The model under review builds one solid part; all positions refer to its coordinate system, in mm. Coordinates: 2 decimals unless noted, no trailing zeros. Write each loop counter-clockwise with the first axis right and the second up, starting at its lowest first coordinate (ties: lowest second). Pieces come first, ordered by that corner, then holes. Notation, with made-up numbers: (27.5, -27.5) - (74.5, -27.5) arc R17 ccw to (74.5, -15.5) - close; hole circle Ø10 at (28, 71.25). An arc over 180 degrees is marked (long way). Put each result on its own line as item: value. Start each with the question number.
Item 1: To check wall thickness, follow L1, parallel to X at y = 2.7, z = 89; L2, parallel to X at y = 1.85, z = 3.5; L3, parallel to Z at x = -77.5, y = 1.85. State the ranges of each line that lie inside material, in increasing order. Write a range as [from, to].
Item 2: For pin 1 (4 mm diameter, centred on x = -82.03, z = 105.37, fed in from +Y); pin 2 (1.8 mm diameter, centred on x = 64.34, z = 87.67, fed in from +Y); pin 3 (1.5 mm diameter, centred on y = 0.5, z = -130.5, fed in from -X); pin 4 (1.5 mm diameter, centred on y = 2, z = -53, fed in from -X), all flat-tipped, find the tip position at first contact; note any pin that passes through.
Item 3: Consider section B-B on z = 167. Give the boundary of the cut face in (x, y).
Item 4: Consider section C-C on x = -133. Give the boundary of the cut face in (y, z).
Item 5: Consider section A-A on y = 1.55. State how many separate pieces and enclosed holes the cut face has, then the cut area to 3 significant figures.
```python
from build123d import *

# Parameters (mm, degrees)
SKETCH1_R           = 200
BOSS_EXTRUDE1_DEPTH = 3
CUT_EXTRUDE1_DEPTH  = 3
SKETCH3_R           = 75
CUT_EXTRUDE2_DEPTH  = 10
SKETCH5_R           = 1.5
CUT_EXTRUDE4_DEPTH  = 73


with BuildPart() as part:
    # Sketch1 → Boss-Extrude1 (new body)
    with BuildSketch(Plane(origin=(0, 0, 0), x_dir=(1, 0, 0), z_dir=(0, 1, 0))):
        with Locations(Location((0, 0, 0), (0, 0, 270))):
            Circle(SKETCH1_R)
    extrude(amount=BOSS_EXTRUDE1_DEPTH)

    # Sketch2 → Cut-Extrude1 (cut)
    with BuildSketch(Plane(origin=(0, 3, 0), x_dir=(1, 0, 0), z_dir=(0, 1, 0))):
        Polygon((-142.885155346, -72.174477228), (-72.174477228, -142.885155346), (-156.069019709, -226.779697828), (-226.779697828, -156.069019709), align=None)
        Polygon((-72.174477228, 142.885155346), (-142.885155346, 72.174477228), (-226.779697828, 156.069019709), (-156.069019709, 226.779697828), align=None)
        Polygon((142.885155346, 72.174477228), (72.174477228, 142.885155346), (156.069019709, 226.779697828), (226.779697828, 156.069019709), align=None)
        Polygon((72.174477228, -142.885155346), (142.885155346, -72.174477228), (226.779697828, -156.069019709), (156.069019709, -226.779697828), align=None)
    extrude(amount=-CUT_EXTRUDE1_DEPTH, mode=Mode.SUBTRACT)

    # Sketch3 → Cut-Extrude2 (cut)
    with BuildSketch(Plane(origin=(0, 3, 0), x_dir=(1, 0, 0), z_dir=(0, 1, 0))):
        with Locations((200, 0)):
            Circle(SKETCH3_R)
    extrude(amount=-CUT_EXTRUDE2_DEPTH, mode=Mode.SUBTRACT)

    # Sketch5 → Cut-Extrude4 (cut)
    with BuildSketch(Plane(origin=(0, 3, 0), x_dir=(1, 0, 0), z_dir=(0, 1, 0))):
        with Locations(Location((82.031457685, -105.365981465, 0), (0, 0, 270))):
            Circle(SKETCH5_R)
        with Locations(Location((64.33964602, -87.674169799, 0), (0, 0, 270))):
            Circle(SKETCH5_R)
        with Locations(Location((105.365981465, -82.031457685, 0), (0, 0, 270))):
            Circle(SKETCH5_R)
        with Locations(Location((87.674169799, -64.33964602, 0), (0, 0, 270))):
            Circle(SKETCH5_R)
        with Locations(Location((-87.674169799, -64.33964602, 0), (0, 0, 270))):
            Circle(SKETCH5_R)
        with Locations(Location((-105.365981465, -82.031457685, 0), (0, 0, 270))):
            Circle(SKETCH5_R)
        with Locations(Location((-82.031457685, -105.365981465, 0), (0, 0, 270))):
            Circle(SKETCH5_R)
        with Locations(Location((-64.33964602, -87.674169799, 0), (0, 0, 270))):
            Circle(SKETCH5_R)
        with Locations(Location((-64.33964602, 87.674169799, 0), (0, 0, 270))):
            Circle(SKETCH5_R)
        with Locations(Location((-82.031457685, 105.365981465, 0), (0, 0, 270))):
            Circle(SKETCH5_R)
        with Locations(Location((-105.365981465, 82.031457685, 0), (0, 0, 270))):
            Circle(SKETCH5_R)
        with Locations(Location((-87.674169799, 64.33964602, 0), (0, 0, 270))):
            Circle(SKETCH5_R)
        with Locations(Location((87.674169799, 64.33964602, 0), (0, 0, 270))):
            Circle(SKETCH5_R)
        with Locations(Location((105.365981465, 82.031457685, 0), (0, 0, 270))):
            Circle(SKETCH5_R)
        with Locations(Location((82.031457685, 105.365981465, 0), (0, 0, 270))):
            Circle(SKETCH5_R)
        with Locations(Location((64.33964602, 87.674169799, 0), (0, 0, 270))):
            Circle(SKETCH5_R)
    extrude(amount=-CUT_EXTRUDE4_DEPTH, mode=Mode.SUBTRACT)


solid = part.part
```
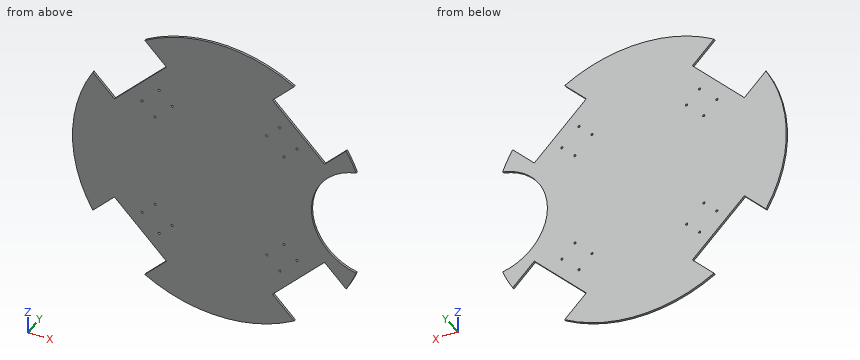
Report:
1. L1: [-179.11, -159.71], [-126.06, -65.04], [-63.64, 63.64], [65.04, 126.06], [159.71, 179.11]
1. L2: [-199.97, 125.08]
1. L3: [-184.37, -148.21], [-137.56, 137.56], [148.21, 184.37]
2. pin 1: y = 3
2. pin 2: through
2. pin 3: x = -85.31
2. pin 4: x = -193.05
3. outline: (-96.29, 0) - (96.29, 0) - (96.29, 3) - (-96.29, 3) - close
4. outline: (0, -82.06) - (3, -82.06) - (3, 82.06) - (0, 82.06) - close
5. separate pieces: 1
5. enclosed holes: 16
5. area: 99,100 mm²
